The model under review builds one solid part; all positions refer to its coordinate system, in mm. Give positions to 0.01 mm unless a question says otherwise; leave off trailing zeros. Loops run counter-clockwise (first coordinate to the right, second up) from the corner with the lowest first, then second, coordinate; pieces in that order, holes last. Notation, with made-up numbers: (70.5, -10.5) - (100.5, -10.5) arc R20 cw to (100.5, 1.5) - close; hole circle Ø3 at (-25, 52). An arc over 180 degrees is marked (long way). Answer as a JSON object with one key per item and string values.
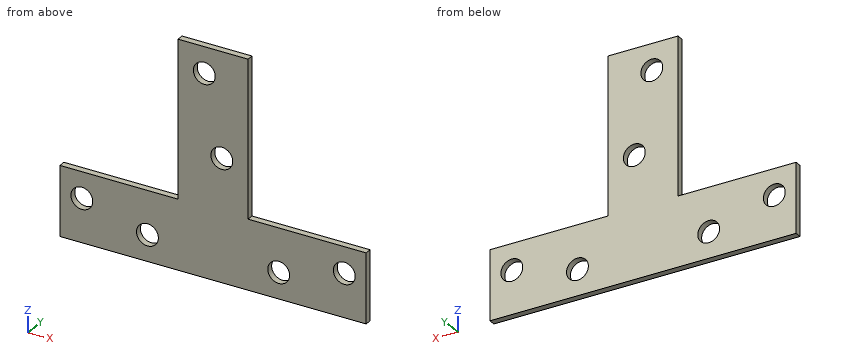
from build123d import *

# Parameters (mm, degrees)
PAD_DEPTH       = 1.5
SKETCH001_R     = 2.5
POCKET_DEPTH    = 126.900362
SKETCH002_R     = 2.5
POCKET001_DEPTH = 1.501


with BuildPart() as part:
    # Sketch → Pad (new body)
    with BuildSketch(Plane.XZ):
        Polygon((0, 0), (35, 0), (35, 16), (8, 16), (8, 52), (0, 52), align=None)
    pad = extrude(amount=PAD_DEPTH)

    # Sketch001 (on Face8 of Pad) → Pocket (cut, through all)
    with BuildSketch(Plane.XZ.offset(1.5)):
        with Locations((30, 10)):
            Circle(SKETCH001_R)
        with Locations((15, 6)):
            Circle(SKETCH001_R)
    pocket = extrude(amount=-POCKET_DEPTH, mode=Mode.SUBTRACT)

    # Mirrored: Pad, Pocket across Sketch V_Axis
    add(pad.mirror(Plane(origin=(0, 0, 0), x_dir=(0, -1, 0), z_dir=(1, 0, 0))))
    add(pocket.mirror(Plane(origin=(0, 0, 0), x_dir=(0, -1, 0), z_dir=(1, 0, 0))), mode=Mode.SUBTRACT)

    # Sketch002 (on Face5 of Mirrored) → Pocket001 (cut, through all)
    with BuildSketch(Plane.XZ.offset(1.5)):
        with Locations((2, 28)):
            Circle(SKETCH002_R)
        with Locations((-2, 46)):
            Circle(SKETCH002_R)
    extrude(amount=-POCKET001_DEPTH, mode=Mode.SUBTRACT)


solid = part.part
Q1. To check wall thickness, follow probe 1 along Z at (x, y) = (-15, -0.5); probe 2 along Z at (x, y) = (-30, -0.85); probe 3 along Z at (x, y) = (-8.5, -1.3). State the ranges of each line that lie inside material, in increasing order. Write a range as [from, to].
Results:
{"probe 1": "z = [0, 3.5], [8.5, 16]", "probe 2": "z = [0, 7.5], [12.5, 16]", "probe 3": "z = [0, 16]"}
Q2. Consider section C-C, the plane z = 10. State the section outline as (x, y) points.
Results:
{"outline": "(-35, -1.5) - (-32.5, -1.5) - (-32.5, 0) - (-35, 0) - close; (-27.5, -1.5) - (27.5, -1.5) - (27.5, 0) - (-27.5, 0) - close; (32.5, -1.5) - (35, -1.5) - (35, 0) - (32.5, 0) - close"}
Q3. Consider section A-A, the plane z = 28. State the section outline as (x, y) points, plus the area to 3 significant figures.
Results:
{"outline": "(-8, -1.5) - (-0.5, -1.5) - (-0.5, 0) - (-8, 0) - close; (4.5, -1.5) - (8, -1.5) - (8, 0) - (4.5, 0) - close", "area": "16.5 mm^2"}
Q4. Clearance check with flat-ended pins moving along their axes: pin 1 Ø0.8 at (y, z) = (-1, 37) entering from +X; pin 2 Ø0.8 at (y, z) = (-0.5, 33.5) entering from -X. State where each tip first meets the part, or that it passes through.
Results:
{"pin 1": "stops at x = 8", "pin 2": "stops at x = -8"}
Q5. Consider section D-D, the plane y = -0.55. State the section outline as (x, z) points.
Results:
{"outline": "(-35, 0) - (35, 0) - (35, 16) - (8, 16) - (8, 52) - (-8, 52) - (-8, 16) - (-35, 16) - close; hole circle Ø5 at (-30, 10); hole circle Ø5 at (-15, 6); hole circle Ø5 at (-2, 46); hole circle Ø5 at (2, 28); hole circle Ø5 at (15, 6); hole circle Ø5 at (30, 10)"}
Q6. Consider section B-B, the plane x = 2. State the section outline as (y, z) points.
Results:
{"outline": "(-1.5, 0) - (0, 0) - (0, 25.5) - (-1.5, 25.5) - close; (-1.5, 30.5) - (0, 30.5) - (0, 52) - (-1.5, 52) - close"}
